```python
from build123d import *

# Parameters (mm, degrees)
F2_R = 5.08
F3_W = 19.05
F3_H = 9.8322601712
F6_D = 10.71626


with BuildPart() as f1:
    # F0 (on Front) → F1 (revolve)
    with BuildSketch(Plane.XZ):
        Polygon((-49.7342673447, 12.7), (-49.7342673447, 0), (49.7342673447, 0), (49.7342673447, 12.7), (28.0643354135, 12.7), (28.0643354135, 32.593707693), (-28.0643354135, 32.593707693), (-28.0643354135, 12.7), align=None)
    revolve(axis=Axis((0, 0, 0), (-1, 0, 0)))

    # F2
    f2_edges = [f1.edges().sort_by_distance(p)[0] for p in [
        (28.064335, 0, -32.593708),
        (-28.064335, 0, -32.593708),
    ]]
    fillet(f2_edges, radius=F2_R)

    # F3 (on Front) → F4 (revolve, cut)
    with BuildSketch(Plane.XZ):
        with Locations((0, 30.0088699144)):
            Rectangle(F3_W, F3_H)
    revolve(axis=Axis((28.0643354135, 0, 0), (-1, 0, 0)), mode=Mode.SUBTRACT)

    # F6 (through all)
    with Locations(Plane.YZ.offset(49.7342673447)):
        with Locations((0, 0)):
            Hole(F6_D / 2)


solid = f1.part
```
Here's how the part is built. I have some questions about the finished solid (model axes, mm). A direction names the side the tool comes from. Coordinates: 2 decimals unless noted, no trailing zeros. Order: outer loops, then holes, each group sorted by start corner. A loop starts at its lowest first (then second) coordinate and runs counter-clockwise, first axis right, second up.
1) We'd pull the mould along Y, two halves only. Please class faces 6 (the face through (0.13, 24.88, -3.27)), 7 (the face through (-0.696, -2.472, -4.754)), 8 (the face through (-49.734, -3, 5)): +Y half, -Y half, draft (parallel to the pull), parting line (faces both ways), or undercut.
2) Will these pins go through, and if not, where does the flat tip stop? pin 1 (12 mm diameter, centred on x = -1, z = 6, fed in from +Y); pin 2 (10 mm diameter, centred on x = 10.5, z = -5, fed in from +Y); pin 3 (3 mm diameter, centred on x = -39.5, y = -10.5, fed in from -Z).
3) Imagine slicing it at C-C on x = -42. List the corners of the cut face in (y, z) for me, and give its area (3 significant figures).
4) I need wall thicknesses on line 1 (X direction, y = 5, z = 26) (3 decimals); line 2 (X direction, y = -8, z = -13.5); line 3 (X direction, y = 7, z = -27.5) (3 decimals). Which ranges of each line are inside material? Lowest first, please.
5) Which directions (+Z, -Z, +X, -X, +Y, -Y) give clear straight access to the entire face, cutting with the end or side of a thin tool? Please do faces 1 (the face through (49.734, -3, -5)), 2 (the face through (16.16, -19.833, -25.865)), 3 (the face through (-28.064, -6, 12)), 4 (the face through (-9.525, -19, -17)), 5 (the face through (28.064, -6, -12)).
6) Imagine slicing it at A-A on z = 0. List the corners of the cut face in (x, y) for me (3 decimals).
Response values:
1. face 6: parting line
1. face 7: undercut
1. face 8: draft
2. pin 1: stops at y = 25.09
2. pin 2: stops at y = 32.59
2. pin 3: stops at z = -8.96
3. outline: circle Ø25.4 at (0, 0); hole circle Ø10.72 at (0, 0)
3. area: 417 mm2
4. line 1: x = -28.064 to -9.525, 9.525 to 28.064
4. line 2: x = -28.06 to 28.06
4. line 3: x = -27.99 to -9.525, 9.525 to 27.99
5. face 1: +Z, -Z, +X, +Y, -Y
5. face 2: +X, -X
5. face 3: -X
5. face 4: none
5. face 5: +X
6. outline: (-49.734, -12.7) - (-28.064, -12.7) - (-28.064, -27.514) arc R5.08 ccw to (-22.984, -32.594) - (-9.525, -32.594) - (-9.525, -25.093) - (9.525, -25.093) - (9.525, -32.594) - (22.984, -32.594) arc R5.08 ccw to (28.064, -27.514) - (28.064, -12.7) - (49.734, -12.7) - (49.734, -5.358) - (-49.734, -5.358) - close; (-49.734, 5.358) - (49.734, 5.358) - (49.734, 12.7) - (28.064, 12.7) - (28.064, 27.514) arc R5.08 ccw to (22.984, 32.594) - (9.525, 32.594) - (9.525, 25.093) - (-9.525, 25.093) - (-9.525, 32.594) - (-22.984, 32.594) arc R5.08 ccw to (-28.064, 27.514) - (-28.064, 12.7) - (-49.734, 12.7) - close
